Work out the finished part from the listing and answer in its coordinate system (mm). A direction names the side the tool comes from. Give positions to 0.01 mm unless a question says otherwise; leave off trailing zeros. Loops run counter-clockwise (first coordinate to the right, second up) from the corner with the lowest first, then second, coordinate; pieces in that order, holes last. Notation, with made-up numbers: M 20,42.25 L 78,42.25 A33 cw 78,79.25 Z; hole C -29.5,86 d8. An arc over 180 degrees is marked long. Use a Markdown table: item, result.
```python
from build123d import *

# Parameters (mm, degrees)
SKETCH_R        = 11
SKETCH_R_2      = 2
PAD_DEPTH       = 11
POCKET_DEPTH    = 7
POCKET001_DEPTH = 1


with BuildPart() as part:
    # Sketch → Pad (new body)
    with BuildSketch(Plane.XY):
        with BuildLine():
            Line((0, -16), (-62.122878, -16))
            Line((-62.122878, -16), (-69.193946, -8.928932))
            Line((-69.193946, -8.928932), (-26.060432, 34.204581))
            Line((-26.060432, 34.204581), (-18.989365, 27.133514))
            Line((-18.989365, 27.133514), (7.04521, 14.36541))
            ThreePointArc((0, -16), (15.585996, -3.616174), (7.04521, 14.36541))
        make_face()
        Circle(SKETCH_R, mode=Mode.SUBTRACT)
        with Locations((-44.091655, 9.102291)):
            Circle(SKETCH_R_2, mode=Mode.SUBTRACT)
    extrude(amount=PAD_DEPTH)

    # Sketch002 → Pocket (cut)
    with BuildSketch(Plane.XY.offset(11)):
        with BuildLine():
            Line((7.04521, 14.36541), (-18.989365, 27.133514))
            Line((-18.989365, 27.133514), (-26.060432, 34.204581))
            Line((-26.060432, 34.204581), (-69.193946, -8.928932))
            Line((-69.193946, -8.928932), (-62.122878, -16))
            Line((-62.122878, -16), (0, -16))
            ThreePointArc((7.04521, 14.36541), (-15.585996, 3.616174), (0, -16))
        make_face()
    extrude(amount=-POCKET_DEPTH, mode=Mode.SUBTRACT)

    # Sketch003 → Pocket001 (cut)
    with BuildSketch(Plane.XY.offset(4)):
        with BuildLine():
            Line((-65.658412, -5.393398), (-58.587344, -12.464466))
            ThreePointArc((-58.587344, -12.464466), (-55.758917, -12.464466), (-55.758917, -9.636039))
            Line((-25.353326, 20.769553), (-55.758917, -9.636039))
            ThreePointArc((-25.353326, 20.769553), (-22.524899, 20.769553), (-22.524899, 23.59798))
            Line((-29.595966, 30.669048), (-22.524899, 23.59798))
            Line((-65.658412, -5.393398), (-29.595966, 30.669048))
        make_face()
    extrude(amount=-POCKET001_DEPTH, mode=Mode.SUBTRACT)


solid = part.part
```
(1) A cutting plane is placed at C-C (y = 12). Write down the section's boundary in (x, z).
Entries:
| item | result |
|---|---|
| outline | M -48.27,0 L 10.58,0 L 10.58,11 L -10.58,11 L -10.58,4 L -34.12,4 L -34.12,3 L -48.27,3 Z |
(2) Consider probe 1 along Y at (x, z) = (0, 5.75); probe 2 along Z at (x, y) = (-35.5, -3.5); probe 3 along X at (y, z) = (-3, 7.5). Determine where each line is inside the solid, lowest interval first. Write a range as [from, to].
Entries:
| item | result |
|---|---|
| probe 1 | y = [-16, -11], [11, 16] |
| probe 2 | z = [0, 4] |
| probe 3 | x = [-15.72, -10.58], [10.58, 15.72] |
(3) The mould has two halves that part along X. Classify faces 1 (the flat face through (-26.11, 27.183, 3.507)), 2 (the flat face through (-22.574, 30.719, 1.972)), 3 (the cylindrical face through (-2.38, -10.74, 5.42)): released by +X, released by -X, zero draft, split by the parting line, or undercut.
Entries:
| item | result |
|---|---|
| face 1 | released by -X |
| face 2 | released by +X |
| face 3 | undercut |
(4) Which of the six approach directions +Z, -Z, +X, -X, +Y, -Y give full straight-line access (tool end or side, diameter ignored) to faces 4 (the flat face through (-47.929, 12.336, 1.528)), 5 (the flat face through (-62.17, -8.88, 3.51)), 6 (the flat face through (-46, 7, 3))?
Entries:
| item | result |
|---|---|
| face 4 | +Z, -Z, -X, +Y |
| face 5 | +Z, +Y |
| face 6 | +Z |
(5) A cutting plane is placed at D-D (x = -57). Write down the section's boundary in (y, z).
Entries:
| item | result |
|---|---|
| outline | M -16,0 L 3.27,0 L 3.27,3 L -13.04,3 L -13.04,4 L -16,4 Z |
(6) Given P1, Ø22, axis at x = -48, y = 0, coming from the +Z side, flat-ended and moving along its own axis, determine where the tip first touches the part or whether it passes through.
Entries:
| item | result |
|---|---|
| P1 | stops at z = 4 |
(7) A cutting plane is placed at A-A (z = 2). Write down the section's boundary in (x, y).
Entries:
| item | result |
|---|---|
| outline | M -69.19,-8.93 L -62.12,-16 L 0,-16 A16 ccw 7.05,14.37 L -18.99,27.13 L -26.06,34.2 Z; hole C -44.09,9.1 d4; hole C 0,0 d22 |
(8) A cutting plane is placed at B-B (y = 2). Write down the section's boundary in (x, z).
Entries:
| item | result |
|---|---|
| outline | M -58.27,0 L -10.82,0 L -10.82,11 L -15.87,11 L -15.87,4 L -44.12,4 L -44.12,3 L -58.27,3 Z; M 10.82,0 L 15.87,0 L 15.87,11 L 10.82,11 Z |
